```python
from build123d import *

# Parameters (mm, degrees)
SKETCH1_R           = 5.08
BOSS_EXTRUDE1_DEPTH = 6.604
SKETCH2_R           = 6.477
CUT_EXTRUDE1_DEPTH  = 3.302
SKETCH3_R           = 75.946
SKETCH3_R_2         = 69.215
CUT_EXTRUDE2_DEPTH  = 1.27
SKETCH4_R           = 2.38125
CUT_EXTRUDE3_DEPTH  = 139.530727768
SKETCH5_R           = 3.77825
CUT_EXTRUDE4_DEPTH  = 1.27
CUT_EXTRUDE5_DEPTH  = 139.530727768
SKETCH10_R          = 57.15
SKETCH10_R_2        = 50.8
CUT_EXTRUDE6_DEPTH  = 1.27
SKETCH12_R          = 2.38125
CUT_EXTRUDE7_DEPTH  = 139.530727768
SKETCH15_R          = 3.175
CUT_EXTRUDE11_DEPTH = 1.27
SKETCH16_W          = 32.206831535
SKETCH16_H          = 125.02997604
SKETCH16_W_2        = 34.902507441
CUT_EXTRUDE12_DEPTH = 139.530727768


with BuildPart() as part:
    # Sketch1 → Boss-Extrude1 (new body)
    with BuildSketch(Plane(origin=(0, 0, 0), x_dir=(0, 0, -1), z_dir=(1, 0, 0))):
        with BuildLine():
            Line((-65.405, -103.855072673), (65.405, -103.855072673))
            ThreePointArc((65.405, -103.855072673), (70.793153673, -101.623226346), (73.025, -96.235072673))
            Line((73.025, -96.235072673), (73.025, -69.997049759))
            ThreePointArc((73.025, -69.997049759), (74.696702219, -57.072253546), (79.601785714, -44.998103417))
            ThreePointArc((79.601785714, -44.998103417), (0, 91.44), (-79.601785714, -44.998103417))
            ThreePointArc((-79.601785714, -44.998103417), (-74.696702219, -57.072253546), (-73.025, -69.997049759))
            Line((-73.025, -69.997049759), (-73.025, -96.235072673))
            ThreePointArc((-73.025, -96.235072673), (-70.793153673, -101.623226346), (-65.405, -103.855072673))
        make_face()
        with Locations(Location((0, 0, 0), (0, 0, 180))):
            Circle(SKETCH1_R, mode=Mode.SUBTRACT)
    extrude(amount=BOSS_EXTRUDE1_DEPTH)

    # Sketch2 → Cut-Extrude1 (cut)
    with BuildSketch(Plane(origin=(0, 0, 0), x_dir=(0, 0, -1), z_dir=(1, 0, 0))):
        with Locations(Location((0, 0, 0), (0, 0, 180))):
            Circle(SKETCH2_R)
    extrude(amount=CUT_EXTRUDE1_DEPTH, mode=Mode.SUBTRACT)

    # Sketch3 → Cut-Extrude2 (cut)
    with BuildSketch(Plane(origin=(6.604, 0, 0), x_dir=(0, 0, -1), z_dir=(1, 0, 0))):
        Circle(SKETCH3_R)
        Circle(SKETCH3_R_2, mode=Mode.SUBTRACT)
    extrude(amount=-CUT_EXTRUDE2_DEPTH, mode=Mode.SUBTRACT)

    # Sketch4 → Cut-Extrude3 (cut, through all)
    with BuildSketch(Plane.ZY):
        with Locations((-66.526040843, 53.05274724)):
            Circle(SKETCH4_R)
        with Locations((0, 85.09)):
            Circle(SKETCH4_R)
        with Locations((-36.919167362, 76.66344097)):
            Circle(SKETCH4_R)
        with Locations((36.919167362, 76.66344097)):
            Circle(SKETCH4_R)
        with Locations((66.526040843, 53.05274724)):
            Circle(SKETCH4_R)
        with Locations((82.956616048, 18.93430627)):
            Circle(SKETCH4_R)
        with Locations((82.956616048, -18.93430627)):
            Circle(SKETCH4_R)
        with Locations((66.526040843, -53.05274724)):
            Circle(SKETCH4_R)
        with Locations((36.919167362, -76.66344097)):
            Circle(SKETCH4_R)
        with Locations((0, -85.09)):
            Circle(SKETCH4_R)
        with Locations((-36.919167361, -76.66344097)):
            Circle(SKETCH4_R)
        with Locations((-66.526040843, -53.05274724)):
            Circle(SKETCH4_R)
        with Locations((-82.956616048, -18.93430627)):
            Circle(SKETCH4_R)
        with Locations((-82.956616048, 18.93430627)):
            Circle(SKETCH4_R)
    extrude(amount=-CUT_EXTRUDE3_DEPTH, mode=Mode.SUBTRACT)

    # Sketch5 → Cut-Extrude4 (cut)
    with BuildSketch(Plane.ZY):
        with Locations((0, 85.09)):
            Circle(SKETCH5_R)
        with Locations((-82.956616048, 18.93430627)):
            Circle(SKETCH5_R)
        with Locations((-66.526040843, 53.05274724)):
            Circle(SKETCH5_R)
        with Locations((36.919167362, 76.66344097)):
            Circle(SKETCH5_R)
        with Locations((-36.919167362, 76.66344097)):
            Circle(SKETCH5_R)
        with Locations((66.526040843, 53.05274724)):
            Circle(SKETCH5_R)
        with Locations((82.956616048, 18.93430627)):
            Circle(SKETCH5_R)
        with Locations((82.956616048, -18.93430627)):
            Circle(SKETCH5_R)
        with Locations((66.526040843, -53.05274724)):
            Circle(SKETCH5_R)
        with Locations((36.919167362, -76.66344097)):
            Circle(SKETCH5_R)
        with Locations((0, -85.09)):
            Circle(SKETCH5_R)
        with Locations((-36.919167362, -76.66344097)):
            Circle(SKETCH5_R)
        with Locations((-66.526040843, -53.05274724)):
            Circle(SKETCH5_R)
        with Locations((-82.956616048, -18.93430627)):
            Circle(SKETCH5_R)
    extrude(amount=-CUT_EXTRUDE4_DEPTH, mode=Mode.SUBTRACT)

    # Sketch9 → Cut-Extrude5 (cut, through all)
    with BuildSketch(Plane.ZY):
        with BuildLine():
            Line((-8.255, 38.60465775), (-8.255, 28.191425558))
            ThreePointArc((-8.255, 28.191425558), (-9.179557622, 24.89186877), (-11.684, 22.553140447))
            ThreePointArc((-11.684, 22.553140447), (-21.997045256, 12.7), (-25.373592562, -1.157929405))
            ThreePointArc((-25.373592562, -1.157929405), (-26.146769513, -4.496204289), (-28.541990702, -6.946673071))
            Line((-28.541990702, -6.946673071), (-37.560114316, -12.153289167))
            ThreePointArc((-37.560114316, -12.153289167), (-43.454984563, -12.392041955), (-47.00205498, -7.677724445))
            ThreePointArc((-47.00205498, -7.677724445), (-41.244459855, 23.8125), (-16.851923077, 44.543835865))
            ThreePointArc((-16.851923077, 44.543835865), (-10.995669144, 43.82914153), (-8.255, 38.60465775))
        make_face()
        with BuildLine():
            Line((8.255, 38.60465775), (8.255, 28.191425558))
            ThreePointArc((8.255, 28.191425558), (9.179557622, 24.89186877), (11.684, 22.553140447))
            ThreePointArc((11.684, 22.553140447), (21.997045256, 12.7), (25.373592562, -1.157929405))
            ThreePointArc((25.373592562, -1.157929405), (26.146769513, -4.496204289), (28.541990702, -6.946673071))
            Line((28.541990702, -6.946673071), (37.560114316, -12.153289167))
            ThreePointArc((37.560114316, -12.153289167), (43.454984563, -12.392041955), (47.00205498, -7.677724445))
            ThreePointArc((47.00205498, -7.677724445), (41.244459855, 23.8125), (16.851923077, 44.543835865))
            ThreePointArc((16.851923077, 44.543835865), (10.995669144, 43.82914153), (8.255, 38.60465775))
        make_face()
        with BuildLine():
            Line((29.305114316, -26.451368583), (20.286990702, -21.244752487))
            ThreePointArc((20.286990702, -21.244752487), (16.967211891, -20.395664481), (13.689592562, -21.395211041))
            ThreePointArc((13.689592562, -21.395211041), (0, -25.4), (-13.689592562, -21.395211041))
            ThreePointArc((-13.689592562, -21.395211041), (-16.967211891, -20.395664481), (-20.286990702, -21.244752487))
            Line((-20.286990702, -21.244752487), (-29.305114316, -26.451368583))
            ThreePointArc((-29.305114316, -26.451368583), (-32.459315419, -31.437099575), (-30.150131903, -36.86611142))
            ThreePointArc((-30.150131903, -36.86611142), (0, -47.625), (30.150131903, -36.86611142))
            ThreePointArc((30.150131903, -36.86611142), (32.459315419, -31.437099575), (29.305114316, -26.451368583))
        make_face()
    extrude(amount=-CUT_EXTRUDE5_DEPTH, mode=Mode.SUBTRACT)

    # Sketch10 → Cut-Extrude6 (cut)
    with BuildSketch(Plane.ZY):
        Circle(SKETCH10_R)
        Circle(SKETCH10_R_2, mode=Mode.SUBTRACT)
    extrude(amount=-CUT_EXTRUDE6_DEPTH, mode=Mode.SUBTRACT)

    # Sketch12 → Cut-Extrude7 (cut, through all)
    with BuildSketch(Plane.ZY):
        with Locations((0, 60.874333344)):
            Circle(SKETCH12_R)
        with Locations((60.874333344, 0)):
            Circle(SKETCH12_R)
        with Locations((0, -60.874333344)):
            Circle(SKETCH12_R)
        with Locations((-60.874333344, 0)):
            Circle(SKETCH12_R)
    extrude(amount=-CUT_EXTRUDE7_DEPTH, mode=Mode.SUBTRACT)

    # Sketch15 → Cut-Extrude11 (cut)
    with BuildSketch(Plane(origin=(6.604, 0, 0), x_dir=(0, 0, -1), z_dir=(1, 0, 0))):
        with Locations((0, 60.874333344)):
            Circle(SKETCH15_R)
        with Locations((60.874333344, 0)):
            Circle(SKETCH15_R)
        with Locations((0, -60.874333344)):
            Circle(SKETCH15_R)
        with Locations((-60.874333344, 0)):
            Circle(SKETCH15_R)
    extrude(amount=-CUT_EXTRUDE11_DEPTH, mode=Mode.SUBTRACT)

    # Sketch16 → Cut-Extrude12 (cut, through all)
    with BuildSketch(Plane.ZY):
        with Locations((-89.128415768, -7.482061739)):
            Rectangle(SKETCH16_W, SKETCH16_H)
        with Locations((90.476253721, -7.482061739)):
            Rectangle(SKETCH16_W_2, SKETCH16_H)
    extrude(amount=-CUT_EXTRUDE12_DEPTH, mode=Mode.SUBTRACT)


solid = part.part
```
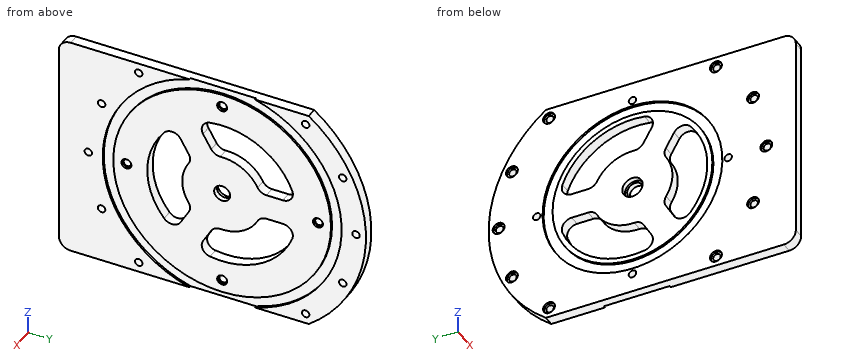
Design review of the part built by this model. Coordinates are the model's own, in mm. Coordinates: 2 decimals unless noted, no trailing zeros. Write each loop counter-clockwise with the first axis right and the second up, starting at its lowest first coordinate (ties: lowest second). Pieces come first, ordered by that corner, then holes.
1) Add section A-A (y = -85.09). Write out the cut boundary in (x, z) (3 decimals), plus the area to 3 significant figures.
2) Insertion check: pin 1 (17 mm diameter, centred on y = 0, z = 0, fed in from -X); pin 2 (2.5 mm diameter, centred on y = -52.5, z = 68, fed in from -X). Each pin has a flat end and moves straight along its axis. Give the tip position at first contact, or say it passes through.
3) Add section D-D (z = 0). State how many separate pieces and enclosed holes the cut face has, plus the area to 3 significant figures.
4) To check wall thickness, follow L1, parallel to Z at x = 4.75, y = -77 (3 decimals); L2, parallel to Y at x = 4.5, z = 10; L3, parallel to Z at x = 6.25, y = -51 (3 decimals). State the ranges of each line that lie inside material, in increasing order.
5) Add section C-C (z = 53.5). Write out the cut boundary in (x, y).
6) Add section B-B (y = 42.5). Write out the cut boundary in (x, z) (3 decimals), plus the area to 3 significant figures.
Check result:
1. outline: (0, -73.025) - (6.604, -73.025) - (6.604, -2.381) - (1.27, -2.381) - (1.27, -3.778) - (0, -3.778) - close; (0, 3.778) - (1.27, 3.778) - (1.27, 2.381) - (6.604, 2.381) - (6.604, 73.025) - (0, 73.025) - close
1. area: 930 mm2
2. pin 1: stops at x = 0
2. pin 2: stops at x = 1.27
3. separate pieces: 7
3. enclosed holes: 0
3. area: 896 mm2
4. L1: z = -73.025 to -39.277, -34.562 to 34.562, 39.277 to 73.025
4. L2: y = -103.86 to -46.56, -23.35 to 23.82, 42.98 to 90.89
4. L3: z = -73.025 to -67.733, -65.319 to -56.274, -46.794 to 46.794, 56.274 to 65.319, 67.733 to 73.025
5. outline: (0, -103.86) - (6.6, -103.86) - (6.6, -53.9) - (5.33, -53.9) - (5.33, -43.91) - (6.6, -43.91) - (6.6, 43.91) - (5.33, 43.91) - (5.33, 53.9) - (6.6, 53.9) - (6.6, 74.16) - (0, 74.16) - (0, 20.1) - (1.27, 20.1) - (1.27, -20.1) - (0, -20.1) - close
6. outline: (0, -73.025) - (6.604, -73.025) - (6.604, -62.941) - (5.334, -62.941) - (5.334, -54.63) - (6.604, -54.63) - (6.604, -21.492) - (0, -21.492) - (0, -27.828) - (1.27, -27.828) - (1.27, -38.208) - (0, -38.208) - close; (0, -9.59) - (6.604, -9.59) - (6.604, 9.59) - (0, 9.59) - close; (0, 21.492) - (6.604, 21.492) - (6.604, 54.63) - (5.334, 54.63) - (5.334, 62.941) - (6.604, 62.941) - (6.604, 73.025) - (0, 73.025) - (0, 38.208) - (1.27, 38.208) - (1.27, 27.828) - (0, 27.828) - close
6. area: 760 mm2
